CAD build for the part. Positions are in the model's coordinates, mm. Coordinates: 2 decimals unless noted, no trailing zeros. Loops run counter-clockwise (first coordinate to the right, second up) from the corner with the lowest first, then second, coordinate; pieces in that order, holes last. Notation, with made-up numbers: (86, 34) -> (124, 34) arc R26 ccw to (124, 73) -> close; hole circle Ø8 at (35.5, 49.25). An arc over 180 degrees is marked (long way). Write each question's results on one line, items separated by ' | '.
from build123d import *

# Parameters (mm, degrees)
SKETCH1_W            = 100
SKETCH1_H            = 100
BOSS_EXTRUDE1_DEPTH  = 100
SKETCH3_R            = 25
CUT_EXTRUDE3_DEPTH   = 151
SKETCH5_R            = 25
CUT_EXTRUDE4_DEPTH   = 151
SKETCH9_R            = 25
CUT_EXTRUDE5_DEPTH   = 100
LPATTERN1_COUNT      = 2
LPATTERN1_PITCH      = 100
LPATTERN1_COUNT_DIR2 = 2
LPATTERN1_PITCH_DIR2 = 100


with BuildPart() as part:
    # Sketch1 → Boss-Extrude1 (new body)
    with BuildSketch(Plane(origin=(0, 0, 0), x_dir=(1, 0, 0), z_dir=(0, 1, 0))):
        Rectangle(SKETCH1_W, SKETCH1_H)
    extrude(amount=BOSS_EXTRUDE1_DEPTH)

    # Sketch3 → Cut-Extrude3 (cut, through all)
    with BuildSketch(Plane.XY.offset(50)):
        with Locations((0, 50)):
            Circle(SKETCH3_R)
    extrude(amount=-CUT_EXTRUDE3_DEPTH, mode=Mode.SUBTRACT)

    # Sketch5 → Cut-Extrude4 (cut, through all)
    with BuildSketch(Plane.ZY.offset(50)):
        with Locations((0, 50)):
            Circle(SKETCH5_R)
    extrude(amount=-CUT_EXTRUDE4_DEPTH, mode=Mode.SUBTRACT)

    # Sketch9 → Cut-Extrude5 (cut)
    with BuildSketch(Plane.ZX.offset(100)):
        with Locations((-50, -50)):
            Circle(SKETCH9_R)
    cut_extrude5 = extrude(amount=-CUT_EXTRUDE5_DEPTH, mode=Mode.SUBTRACT)

    # LPattern1: Cut-Extrude5 2 × 2
    with Locations(*[(i * LPATTERN1_PITCH, 0, j * LPATTERN1_PITCH_DIR2) for i in range(LPATTERN1_COUNT) for j in range(LPATTERN1_COUNT_DIR2) if (i, j) != (0, 0)]):
        add(cut_extrude5, mode=Mode.SUBTRACT)


solid = part.part
1) Slice it at B-B (y = 59). Write the cut outline in (x, z), then the cut area to 3 significant figures.
Outcome:
outline: (-50, -25) arc R25 cw to (-25, -50) -> (-23.32, -50) -> (-23.32, -23.32) -> (-50, -23.32) -> close; (-50, 23.32) -> (-23.32, 23.32) -> (-23.32, 50) -> (-25, 50) arc R25 cw to (-50, 25) -> close; (23.32, -50) -> (25, -50) arc R25 cw to (50, -25) -> (50, -23.32) -> (23.32, -23.32) -> close; (23.32, 23.32) -> (50, 23.32) -> (50, 25) arc R25 cw to (25, 50) -> (23.32, 50) -> close | area: 883 mm^2
2) Pin check, flat tips, straight feed: pin 1 (10 mm diameter, centred on x = 33, y = 48, fed in from +Z); pin 2 (10 mm diameter, centred on y = 58, z = -34, fed in from -X). Stop position of each tip, or through.
Outcome:
pin 1: stops at z = 38.13 | pin 2: stops at x = -36.44
3) Two-plate mould, pull along Y, no slides. Class faces 1 (the flat face through (-1, 100, -1)), 2 (the cylindrical face through (30.206, 57.509, 23.846)), 3 (the cylindrical face through (23.846, 57.509, -30.206)), 4 (the flat face through (-50, 86, 0)): pulls with the +Y half, pulls with the -Y half, needs draft (parallel to the pull), parting line crosses it, or undercut.
Outcome:
face 1: pulls with the +Y half | face 2: undercut | face 3: undercut | face 4: needs draft
4) Slice it at D-D (y = 92.5). Write the cut outline in (x, z).
Outcome:
outline: (-50, -25) arc R25 cw to (-25, -50) -> (25, -50) arc R25 cw to (50, -25) -> (50, 25) arc R25 cw to (25, 50) -> (-25, 50) arc R25 cw to (-50, 25) -> close
5) Slice it at C-C (x = 4.5). Write the cut outline in (y, z).
Outcome:
outline: (0, -50) -> (25.41, -50) -> (25.41, -4.5) arc R25 cw to (25.41, 4.5) -> (25.41, 50) -> (0, 50) -> close; (74.59, -50) -> (100, -50) -> (100, 50) -> (74.59, 50) -> (74.59, 4.5) arc R25 cw to (74.59, -4.5) -> close
6) Slice it at A-A (z = -13.5). Write the cut outline in (x, y), then the cut area to 3 significant figures.
Outcome:
outline: (-50, 0) -> (50, 0) -> (50, 28.96) -> (13.5, 28.96) arc R25 cw to (-13.5, 28.96) -> (-50, 28.96) -> close; (-50, 71.04) -> (-13.5, 71.04) arc R25 cw to (13.5, 71.04) -> (50, 71.04) -> (50, 100) -> (-50, 100) -> close | area: 5,650 mm^2
7) Drill centre lines: L1, parallel to Y at x = -1, z = 8; L2, parallel to Z at x = -32.5, y = 35; L3, parallel to Z at x = -28, y = 50. Where is each one in solid material? Low to high. Write a range as from..to.
Outcome:
L1: y = 0..25.02, 74.98..100 | L2: z = -32.15..-20, 20..32.15 | L3: z = -38.13..-25, 25..38.13
